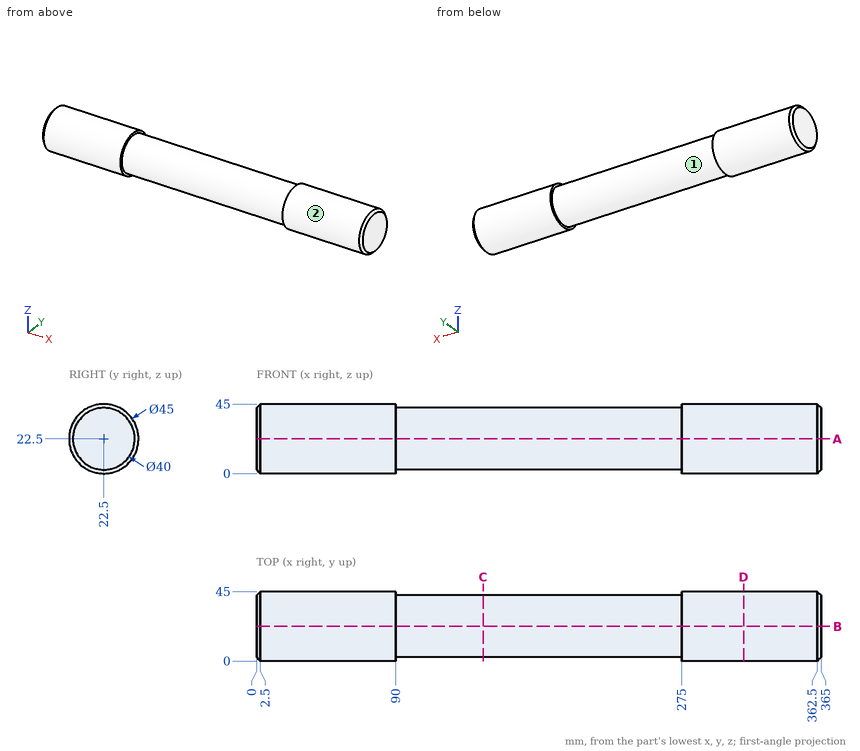
Geometry: see drawing. Coordinates: mm, zero at the bounding-box minimum. A direction names the side the tool comes from. Coordinates: 2 decimals unless noted, no trailing zeros. Loops run counter-clockwise (first coordinate to the right, second up) from the corner with the lowest first, then second, coordinate; pieces in that order, holes last. Notation, with made-up numbers: M -19,80 L 26,80 A20 ccw 26,109 Z; hole C 33.5,-30 d10. An arc over 180 degrees is marked long. Put each result on its own line as item: value. Start each with the question number.
1) Cut plane D-D on x = 315. Return the cut outline in (y, z).
2) Ray query, L1, parallel to X at y = 31, z = 3.5; L2, parallel to X at y = 40, z = 35; L3, parallel to Y at x = 136, z = 22. Return the intervals inside material, ascending. Write a range as from..to.
3) Contact query for flat-ended pins moving along their axis: pin 1 Ø10 at (x, y) = (229.5, 12.5) entering from -Z; pin 2 Ø1.5 at (x, z) = (258.5, 23.5) entering from +Y; pin 3 Ø3 at (x, z) = (276, 4.5) entering from +Y. Output: stop coordinate, or through.
4) Cut plane C-C on x = 146.5. Return the cut outline in (y, z), then the cut area to 3 significant figures.
5) Cut plane A-A on z = 22.5. Return the cut outline in (x, y), then the cut area to 3 significant figures.
6) Reachability of the marked faces 1 and 2 from +Z, -Z, +X, -X, +Y, -Y: full face, straight path, thin tool, end or side. Return the list, or none.
The answers:
1. outline: C 22.5,22.5 d45
2. L1: x = 0.81..90, 275..364.19
2. L2: x = 1.51..90, 275..363.49
2. L3: y = 2.51..42.49
3. pin 1: stops at z = 3.14
3. pin 2: stops at y = 42.5
3. pin 3: stops at y = 37.8
4. outline: C 22.5,22.5 d40
4. area: 1,260 mm²
5. outline: M 0,2.5 L 2.5,0 L 90,0 L 90,2.5 L 275,2.5 L 275,0 L 362.5,0 L 365,2.5 L 365,42.5 L 362.5,45 L 275,45 L 275,42.5 L 90,42.5 L 90,45 L 2.5,45 L 0,42.5 Z
5. area: 15,500 mm²
6. face 1: none
6. face 2: +X, -X
